The listing builds one solid part. Answer for the finished solid, in the listing's coordinates (mm). Give positions to 0.01 mm unless a question says otherwise; leave off trailing zeros. Write each loop counter-clockwise with the first axis right and the second up, starting at its lowest first coordinate (ties: lowest second). Pieces come first, ordered by that corner, then holes. Notation, with made-up numbers: (69, 76) - (113, 76) arc R22 cw to (113, 95) - close; hole circle Ø11 at (-11, -20). An arc over 180 degrees is marked (long way). One line per question, with ' | ' between items. Start each with the question number.
1. Given P1, Ø5.5, axis at x = 7, y = -75.5, coming from the +Z side; P2, Ø2.5, axis at x = 8.5, z = -45.5, coming from the +Y side; P3, Ø5, axis at x = 3, z = 16, coming from the -Y side, each flat-ended and moving along its own axis, determine where each tip first touches the part or whether it passes through.
2. A cutting plane is placed at B-B (y = 132). Determine the outline of the cut face in (x, z), then the cut area to 3 significant figures.
3. Find the intervals of material crossed by L1, parallel to Z at x = 8, y = -141; L2, parallel to Y at x = 8.5, z = 22; L3, parallel to Z at x = 4.5, y = -76.5, in increasing order. Write a range as from..to.
4. A cutting plane is placed at A-A (z = 7). Determine the outline of the cut face in (x, y), then the cut area to 3 significant figures.
```python
from build123d import *

# Parameters (mm, degrees)
SKETCH_W     = 440
SKETCH_H     = 300
PAD_DEPTH    = 10
PAD001_DEPTH = 8
POCKET_DEPTH = 5
CHAMFER_SIZE = 5


with BuildPart() as part:
    # Sketch → Pad (new body)
    with BuildSketch(Plane.YZ):
        Rectangle(SKETCH_W, SKETCH_H)
        with BuildLine():
            Line((-195, 110), (-195, -110))
            ThreePointArc((-195, -110), (-190.606602, -120.606602), (-180, -125))
            Line((-180, -125), (180, -125))
            ThreePointArc((180, -125), (190.606602, -120.606602), (195, -110))
            Line((195, -110), (195, 110))
            ThreePointArc((195, 110), (190.606602, 120.606602), (180, 125))
            Line((180, 125), (-180, 125))
            ThreePointArc((-180, 125), (-190.606602, 120.606602), (-195, 110))
        make_face(mode=Mode.SUBTRACT)
    extrude(amount=PAD_DEPTH)

    # Sketch001 (on Face14 of Pad) → Pad001 (join)
    with BuildSketch(Plane.YZ.offset(10)):
        with BuildLine():
            Line((-240, 130), (-240, -130))
            ThreePointArc((-240, -130), (-228.284271, -158.284271), (-200, -170))
            Line((-200, -170), (200, -170))
            ThreePointArc((200, -170), (228.284271, -158.284271), (240, -130))
            Line((240, -130), (240, 130))
            ThreePointArc((240, 130), (228.284271, 158.284271), (200, 170))
            Line((200, 170), (-200, 170))
            ThreePointArc((-200, 170), (-228.284271, 158.284271), (-240, 130))
        make_face()
        with BuildLine():
            Line((-215, 115), (-215, -115))
            ThreePointArc((-215, -115), (-206.213203, -136.213203), (-185, -145))
            Line((-185, -145), (185, -145))
            ThreePointArc((185, -145), (206.213203, -136.213203), (215, -115))
            Line((215, -115), (215, 115))
            ThreePointArc((215, 115), (206.213203, 136.213203), (185, 145))
            Line((185, 145), (-185, 145))
            ThreePointArc((-185, 145), (-206.213203, 136.213203), (-215, 115))
        make_face(mode=Mode.SUBTRACT)
    extrude(amount=PAD001_DEPTH)

    # Sketch002 (on Face23 of Pad001) → Pocket (cut)
    with BuildSketch(Plane.YZ.offset(10)):
        with BuildLine():
            Line((-208, 113), (-208, -113))
            ThreePointArc((-208, -113), (-200.67767, -130.67767), (-183, -138))
            Line((-183, -138), (183, -138))
            ThreePointArc((183, -138), (200.67767, -130.67767), (208, -113))
            Line((208, -113), (208, 113))
            ThreePointArc((208, 113), (200.67767, 130.67767), (183, 138))
            Line((183, 138), (-183, 138))
            ThreePointArc((-183, 138), (-200.67767, 130.67767), (-208, 113))
        make_face()
        with BuildLine():
            Line((-203, 113), (-203, -113))
            ThreePointArc((-203, -113), (-197.142136, -127.142136), (-183, -133))
            Line((-183, -133), (183, -133))
            ThreePointArc((183, -133), (197.142136, -127.142136), (203, -113))
            Line((203, -113), (203, 113))
            ThreePointArc((203, 113), (197.142136, 127.142136), (183, 133))
            Line((183, 133), (-183, 133))
            ThreePointArc((-183, 133), (-197.142136, 127.142136), (-203, 113))
        make_face(mode=Mode.SUBTRACT)
    extrude(amount=-POCKET_DEPTH, mode=Mode.SUBTRACT)

    # Chamfer
    chamfer_edges = [part.edges().sort_by_distance(p)[0] for p in [
        (18, -240, 0),
        (18, -228.284271, 158.284271),
        (18, 0, 170),
        (18, -228.284271, -158.284271),
        (18, 0, -170),
        (18, 240, 0),
        (18, 228.284271, -158.284271),
        (18, 228.284271, 158.284271),
    ]]
    chamfer(chamfer_edges, length=CHAMFER_SIZE)


solid = part.part
```
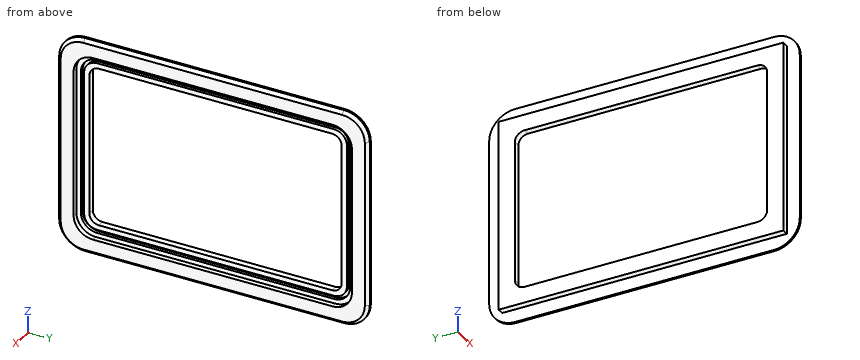
Determined:
1) P1: z = 150 | P2: y = 220 | P3: y = -220
2) outline: (0, -150) - (10, -150) - (10, -170) - (13, -170) - (18, -165) - (18, -145) - (10, -145) - (10, -138) - (5, -138) - (5, -133) - (10, -133) - (10, -125) - (0, -125) - close; (0, 125) - (10, 125) - (10, 133) - (5, 133) - (5, 138) - (10, 138) - (10, 145) - (18, 145) - (18, 165) - (13, 170) - (10, 170) - (10, 150) - (0, 150) - close | area: 825 mm2
3) L1: -150..-138, -133..-125, 125..133, 138..150 | L2: -220..-208, -203..-195, 195..203, 208..220 | L3: -150..-125, 125..150
4) outline: (0, -220) - (10, -220) - (10, -240) - (13, -240) - (18, -235) - (18, -215) - (10, -215) - (10, -208) - (5, -208) - (5, -203) - (10, -203) - (10, -195) - (0, -195) - close; (0, 195) - (10, 195) - (10, 203) - (5, 203) - (5, 208) - (10, 208) - (10, 215) - (18, 215) - (18, 235) - (13, 240) - (10, 240) - (10, 220) - (0, 220) - close | area: 825 mm2
